from build123d import *

# Parameters (mm, degrees)
F3_DEPTH  = 4
F5_DEPTH  = 1
F6_R      = 3.25
F7_DEPTH  = 4
F8_W      = 118.9
F8_H      = 69.5
F9_DEPTH  = 0.8
F10_R     = 5
F11_D     = 2.6
F11_DEPTH = 4.001
F12_SIZE  = 2.99999
F13_SIZE  = 1
F14_D     = 3.5


# Not quite as in the source:
# - a fillet or chamfer is up to 0.001 mm smaller than in the source, because OpenCascade refuses the exact size
# - after a boolean that leaves OpenCascade's solid faulty, fix() repairs it


with BuildPart() as f3:
    # F2 (on Top) → F3 (new body)
    with BuildSketch(Plane.XY):
        with BuildLine():
            Line((12, 31.5), (-12, 31.5))
            ThreePointArc((-12, 31.5), (-13.4142135624, 30.9142135624), (-14, 29.5))
            Line((-14, 29.5), (-14, -29.5))
            ThreePointArc((-14, -29.5), (-13.4142135624, -30.9142135624), (-12, -31.5))
            Line((-12, -31.5), (12, -31.5))
            ThreePointArc((12, -31.5), (13.4142135624, -30.9142135624), (14, -29.5))
            Line((14, -29.5), (14, 29.5))
            ThreePointArc((14, 29.5), (13.4142135624, 30.9142135624), (12, 31.5))
        make_face()
        with BuildLine():
            ThreePointArc((10, -23), (9.4142135624, -24.4142135624), (8, -25))
            Line((8, -25), (-8, -25))
            ThreePointArc((-8, -25), (-9.4142135624, -24.4142135624), (-10, -23))
            Line((-10, -23), (-10, 23))
            ThreePointArc((-10, 23), (-9.4142135624, 24.4142135624), (-8, 25))
            Line((-8, 25), (8, 25))
            ThreePointArc((8, 25), (9.4142135624, 24.4142135624), (10, 23))
            Line((10, 23), (10, -23))
        make_face(mode=Mode.SUBTRACT)
    extrude(amount=F3_DEPTH)

    # F4 (on Top) → F5 (join)
    with BuildSketch(Plane.XY):
        with BuildLine():
            ThreePointArc((100.65, 26.5), (100.3571067812, 27.2071067812), (99.65, 27.5))
            Line((99.65, 27.5), (14, 27.5))
            ThreePointArc((14, 27.5), (13, 26.5), (14, 25.5))
            Line((14, 25.5), (25.65, 25.5))
            Line((25.65, 25.5), (25.65, -25.5))
            Line((25.65, -25.5), (14, -25.5))
            ThreePointArc((14, -25.5), (13, -26.5), (14, -27.5))
            Line((14, -27.5), (99.65, -27.5))
            ThreePointArc((99.65, -27.5), (100.3571067812, -27.2071067812), (100.65, -26.5))
            Line((100.65, -26.5), (100.65, 26.5))
        make_face()
        with BuildLine():
            Line((64.3250247719, -2.0888654384), (96.5705497341, -25.5))
            Line((96.5705497341, -25.5), (29.7294502659, -25.5))
            Line((29.7294502659, -25.5), (61.9749752281, -2.0888654384))
            ThreePointArc((61.9749752281, -2.0888654384), (63.15, -1.7072957846), (64.3250247719, -2.0888654384))
        make_face(mode=Mode.SUBTRACT)
        with BuildLine():
            Line((59.218749446, -1.6184303462), (27.65, -24.5382073412))
            Line((27.65, -24.5382073412), (27.65, 24.5382073412))
            Line((27.65, 24.5382073412), (59.218749446, 1.6184303462))
            ThreePointArc((59.218749446, 1.6184303462), (60.0437246741, 0), (59.218749446, -1.6184303462))
        make_face(mode=Mode.SUBTRACT)
        with BuildLine():
            Line((61.9749752281, 2.0888654384), (29.7294502659, 25.5))
            Line((29.7294502659, 25.5), (96.5705497341, 25.5))
            Line((96.5705497341, 25.5), (64.3250247719, 2.0888654384))
            ThreePointArc((64.3250247719, 2.0888654384), (63.15, 1.7072957846), (61.9749752281, 2.0888654384))
        make_face(mode=Mode.SUBTRACT)
        with BuildLine():
            Line((67.081250554, 1.6184303462), (98.65, 24.5382073412))
            Line((98.65, 24.5382073412), (98.65, -24.5382073412))
            Line((98.65, -24.5382073412), (67.081250554, -1.6184303462))
            ThreePointArc((67.081250554, -1.6184303462), (66.2562753259, 0), (67.081250554, 1.6184303462))
        make_face(mode=Mode.SUBTRACT)
    extrude(amount=F5_DEPTH)

    # F6 (on face) → F7 (join)
    with BuildSketch(Plane(origin=(0, 0, 0), x_dir=(1, 0, 0), z_dir=(0, 0, -1))):
        with Locations((-5.65, -31.5)):
            Circle(F6_R)
        with Locations((-5.65, 31.5)):
            Circle(F6_R)
        with Locations((99.65, 26.5)):
            Circle(F6_R)
        with Locations((99.65, -26.5)):
            Circle(F6_R)
        with Locations((26.65, -26.5)):
            Circle(F6_R)
        with Locations((26.65, 26.5)):
            Circle(F6_R)
    extrude(amount=-F7_DEPTH)

    # F8 (on Top) → F9 (join)
    with BuildSketch(Plane.XY):
        with Locations((45.45, 0)):
            Rectangle(F8_W, F8_H)
    extrude(amount=-F9_DEPTH)

    # F10
    f10_edges = [f3.edges().sort_by_distance(p)[0] for p in [
        (-14, -34.75, -0.4),
        (-14, 34.75, -0.4),
        (104.9, 34.75, -0.4),
        (104.9, -34.75, -0.4),
    ]]
    fillet(f10_edges, radius=F10_R)

    # F11 (through all, one way)
    with BuildSketch(Plane(origin=(0, 0, 0), x_dir=(1, 0, 0), z_dir=(0, 0, -1))):
        with Locations((99.65, -26.5), (26.65, -26.5), (-5.65, -31.5), (-5.65, 31.5), (26.65, 26.5), (99.65, 26.5)):
            Circle(F11_D / 2)
    extrude(amount=-F11_DEPTH, mode=Mode.SUBTRACT)

    # F12 (size 3 in the source; OpenCascade refuses exactly that, so slightly less here)
    f12_edges = [f3.edges().sort_by_distance(p)[0] for p in [
        (29.279949, -24.590585, 1),
        (29.279949, 24.590585, 1),
        (97.020051, -24.590585, 1),
        (14, -26.5, 1),
        (14, 26.5, 1),
        (29.86034, -27.006177, 1),
        (23.4, -26.5, 1),
        (26.65, -23.25, 1),
        (29.86034, -25.993823, 1),
        (96.4, -26.5, 1),
        (99.65, -23.25, 1),
        (29.86034, 25.993823, 1),
        (26.65, 23.25, 1),
        (23.4, 26.5, 1),
        (29.86034, 27.006177, 1),
        (99.65, 23.25, 1),
    ]]
    chamfer(f12_edges, length=F12_SIZE)

    # F13
    f13_edges = [f3.edges().sort_by_distance(p)[0] for p in [
        (24.351903, 24.201903, 0),
        (28.125957, 23.604478, 0),
        (26.65, 29.75, 0),
        (26.65, -29.75, 0),
        (24.351903, -24.201903, 0),
        (28.125957, -23.604478, 0),
        (102.277975, -24.587868, 0),
        (98.174043, -23.604478, 0),
        (100.156177, 29.71034, 0),
        (98.174043, 23.604478, 0),
        (100.156177, -29.71034, 0),
        (102.277975, 24.587868, 0),
    ]]
    chamfer(f13_edges, length=F13_SIZE)

    # F14 (through all)
    with Locations(Plane.XY):
        with Locations((0, 0), (43.9, 0), (82.4, 0)):
            Hole(F14_D / 2)

    add(f3.part.fix(), mode=Mode.REPLACE)


solid = f3.part
For this review, take the finished solid that the model builds, in its own axes (mm). Round coordinates to 2 decimals unless told otherwise and drop trailing zeros. Loops run counter-clockwise (first coordinate to the right, second up) from the corner with the lowest first, then second, coordinate; pieces in that order, holes last. Notation, with made-up numbers: (72, -23.5) - (122, -23.5) arc R19 cw to (122, -9.5) - close; hole circle Ø5 at (-14, -3). An arc over 180 degrees is marked (long way). One line per question, with ' | ' between items.
Q1. For line 1 along Y through (x, z) = (-5.65, 1.7); line 2 along Y through (x, z) = (-4.5, 3.35); line 3 along Y through (x, z) = (63, 0.75), list the stretches that pass through material, from the lowest coordinate up. Write a range as [from, to].
Taken from the geometry:
line 1: y = [-34.75, -32.8], [-30.2, -25], [25, 30.2], [32.8, 34.75] | line 2: y = [-34.54, -32.11], [-30.89, -25], [25, 30.89], [32.11, 34.54] | line 3: y = [-27.5, -25.5], [-1.71, 1.71], [25.5, 27.5]
Q2. For pin 1 (1.6 mm diameter, centred on x = 26.65, y = 26.5, fed in from +Z); pin 2 (3 mm diameter, centred on x = 27, y = 27, fed in from +Z); pin 3 (1 mm diameter, centred on x = 99.5, y = 1, fed in from +Z); pin 4 (2 mm diameter, centred on y = -0.5, z = 2.5, fed in from +X), all flat-tipped, find the tip position at first contact; note any pin that passes through.
Taken from the geometry:
pin 1: stops at z = 0 | pin 2: stops at z = 4 | pin 3: stops at z = 1 | pin 4: stops at x = 14
Q3. Take a section at D-D (y = -8). Give the boundary of the cut face in (x, z).
Taken from the geometry:
outline: (-14, -0.8) - (104.9, -0.8) - (104.9, 0) - (100.65, 0) - (100.65, 1) - (98.65, 1) - (98.65, 0) - (75.87, 0) - (75.87, 1) - (72.47, 1) - (72.47, 0) - (53.83, 0) - (53.83, 1) - (50.43, 1) - (50.43, 0) - (27.65, 0) - (27.65, 1) - (25.65, 1) - (25.65, 0) - (14, 0) - (14, 4) - (10, 4) - (10, 0) - (-10, 0) - (-10, 4) - (-14, 4) - close
Q4. The part is to be moulded in two halves that separate along X. For faces 1 (the flat face through (62, -28, 0)), 2 (the cylindrical face through (-5.72, 34.75, 1.97)), 3 (the flat face through (5, -31.5, 2)), say which applies: released by +X, released by -X, zero draft, split by the parting line, or undercut.
Taken from the geometry:
face 1: undercut | face 2: split by the parting line | face 3: zero draft
Q5. Take a section at B-B (x = 0). Give the boundary of the cut face in (y, z).
Taken from the geometry:
outline: (-34.75, -0.8) - (-1.75, -0.8) - (-1.75, 0) - (-25, 0) - (-25, 4) - (-31.5, 4) - (-31.5, 0) - (-34.75, 0) - close; (1.75, -0.8) - (34.75, -0.8) - (34.75, 0) - (31.5, 0) - (31.5, 4) - (25, 4) - (25, 0) - (1.75, 0) - close
Q6. Take a section at A-A (y = 0). State how many separate pieces and enclosed holes the cut face has, and give its area (3 significant figures).
Taken from the geometry:
separate pieces: 4 | enclosed holes: 0 | area: 129 mm²
